```python
from build123d import *

# Parameters (mm, degrees)
FILLET1_R                = 2.5
CIRPATTERN1_COUNT        = 4
FILLET1_OF_CIRPATTERN1_R = 2.5
SKETCH3_W                = 9
SKETCH3_H                = 9
CUT_EXTRUDE1_DEPTH       = 11
SKETCH4_R                = 7.5
CUT_EXTRUDE2_DEPTH       = 3
CUT_EXTRUDE3_REACH       = 53.176
SKETCH5_R                = 2


with BuildPart() as part:
    # Sketch1 → Revolve1 (revolve)
    with BuildSketch(Plane(origin=(0, 0, 0), x_dir=(0, 0, -1), z_dir=(1, 0, 0)), mode=Mode.PRIVATE) as revolve1_sk:
        with BuildLine():
            Line((0, -8), (0, 8))
            Line((0, 8), (-9.68857754, 8))
            ThreePointArc((-9.68857754, 8), (-12, 0), (-9.68857754, -8))
            Line((-9.68857754, -8), (0, -8))
        make_face()
    revolve(revolve1_sk.sketch.rotate(Axis((0, 0, 0), (0, 1, 0)), 180), axis=Axis((0, 0, 0), (0, 1, 0)))

    # Sketch2 → Revolve2 (revolve)
    with BuildSketch(Plane.XY, mode=Mode.PRIVATE) as revolve2_sk:
        with BuildLine():
            Line((0, 0), (-35, 0))
            ThreePointArc((-35, 0), (-32.975720289, -4.493734325), (-28.26878394, -5.95527691))
            Line((-28.26878394, -5.95527691), (0, -2.484306687))
            Line((0, -2.484306687), (0, 0))
        make_face()
    revolve2 = revolve(revolve2_sk.sketch.rotate(Axis((0, 0, 0), (-1, 0, 0)), 341.200414784), axis=Axis((0, 0, 0), (-1, 0, 0)))

    # Fillet1
    fillet1_edges = [part.edges().sort_by_distance(p)[0] for p in [
        (-11.471875359, 3.685197146, 1.254513651),
    ]]
    fillet(fillet1_edges, radius=FILLET1_R)

    # CirPattern1: Revolve2 ×4 about axis
    cirpattern1_axis = Axis((0, 8, 0), (0, -1, 0))
    for i in range(1, CIRPATTERN1_COUNT):
        add(revolve2.rotate(cirpattern1_axis, i * 360 / CIRPATTERN1_COUNT))

    # Fillet1 of CirPattern1
    fillet1_of_cirpattern1_edges = [part.edges().sort_by_distance(p)[0] for p in [
        (-1.254513651, 3.685197146, -11.471875359),
        (11.471875359, 3.685197146, -1.254513651),
        (1.254513651, 3.685197146, 11.471875359),
    ]]
    fillet(fillet1_of_cirpattern1_edges, radius=FILLET1_OF_CIRPATTERN1_R)

    # Sketch3 → Cut-Extrude1 (cut)
    with BuildSketch(Plane(origin=(0, 8, 0), x_dir=(1, 0, 0), z_dir=(0, 1, 0))):
        Rectangle(SKETCH3_W, SKETCH3_H)
    extrude(amount=-CUT_EXTRUDE1_DEPTH, mode=Mode.SUBTRACT)

    # Sketch4 → Cut-Extrude2 (cut)
    with BuildSketch(Plane.XZ.offset(8)):
        with Locations(Location((0, 0, 0), (0, 0, 270))):
            Circle(SKETCH4_R)
    extrude(amount=-CUT_EXTRUDE2_DEPTH, mode=Mode.SUBTRACT)

    # Sketch5 → Cut-Extrude3 (cut, up to next)
    with BuildSketch(Plane.XZ.offset(5), mode=Mode.PRIVATE) as cut_extrude3_sk1:
        with Locations(Location((0, 0, 0), (0, 0, 270))):
            Circle(SKETCH5_R)
    cut_extrude3_tool1 = extrude(cut_extrude3_sk1.sketch, amount=-CUT_EXTRUDE3_REACH, mode=Mode.PRIVATE) & part.part
    add(cut_extrude3_tool1.solids().sort_by_distance((0, -5, 0))[0], mode=Mode.SUBTRACT)


solid = part.part
```
Verification items for the finished model (mm, model axes). A direction names the side the tool comes from. Round coordinates to 2 decimals unless told otherwise and drop trailing zeros. Order: outer loops, then holes, each group sorted by start corner. A loop starts at its lowest first (then second) coordinate and runs counter-clockwise, first axis right, second up. Notation, with made-up numbers: (85, 37.25) - (97, 37.25) arc R23 cw to (97, 61.25) - close; hole circle Ø2 at (-29.5, 27.5). An arc over 180 degrees is marked (long way). Use CSV: the item, a comma, the result in double quotes. Start each with the question number.
1) Access from +Z, -Z, +X, -X, +Y, -Y to the whole of each face (thin tool, end or side, straight path). Record for faces 1 (the cylindrical face through (0.33, -6.521, 7.493)), 2 (the flat face through (0, 3, -4.5)), 3 (the conical face through (20.638, -5.017, 0.116)), 4 (the cylindrical face through (-2, -4, 0)), 5 (the flat face through (6, 8, 0)).
2) Section check B-B, the plane z = 21.5. Record the cut outline in (x, y).
3) Thickness scan on L1, parallel to X at y = -6.7, z = 0; L2, parallel to X at y = -3.55, z = 0; L3, parallel to Z at x = 3, y = -1. Record the ranges inside material, lowest first.
4) Mould release check, pull along X, two halves, no side actions. Record for faces 6 (the flat face through (-2, -5, -2)), 7 (the conical face through (-20.638, 4.754, -1.607)), 8 (the conical face through (4.287, 2.609, -20.637)), 9 (the flat face through (6, -8, -5)): +X half, -X half, draft (parallel to the pull), parting line (faces both ways), or undercut.
5) Section check A-A, the plane x = 17. Record the cut outline in (y, z), plus the area to 3 significant figures.
6) Go/stop test with flat-tipped pins: P1, Ø2, axis at y = -5, z = -16.5, coming from the +X side; P2, Ø4, axis at y = -1.5, z = -27.5, coming from the -X side; P3, Ø5, axis at x = 22.5, z = -5, coming from the -Y side. Record where each tip stops, or that it passes through.
Answers:
1,face 1,"-Y"
1,face 2,"+Y"
1,face 3,"none"
1,face 4,"+Y, -Y"
1,face 5,"+Z, -Z, +X, -X, +Y"
2,outline,"circle Ø10.25 at (0, 0)"
3,L1,"x = -10.42 to -7.5, 7.5 to 10.42"
3,L2,"x = -33.84 to -2, 2 to 33.84"
3,L3,"z = -34.1 to -4.5, 4.5 to 34.1"
4,face 6,"undercut"
4,face 7,"undercut"
4,face 8,"parting line"
4,face 9,"draft"
5,outline,"circle Ø9.14 at (0, 0)"
5,area,"65.7 mm²"
6,P1,"stops at x = 2.1"
6,P2,"stops at x = -6"
6,P3,"stops at y = -4.66"
